Here's how the part is built. I have some questions about the finished solid (model axes, mm). A direction names the side the tool comes from. Round coordinates to 2 decimals unless told otherwise and drop trailing zeros. Write each loop counter-clockwise with the first axis right and the second up, starting at its lowest first coordinate (ties: lowest second). Pieces come first, ordered by that corner, then holes. Notation, with made-up numbers: (69, 10) -> (81, 10) arc R12 ccw to (81, 19) -> close; hole circle Ø4 at (-28.5, 63.5). An arc over 180 degrees is marked (long way). Put each result on its own line as item: value. Start each with the question number.
1. Suppose I cut it at C-C (x = 0). Please give me the cut outline in (y, z), then the cut area to 3 significant figures.
2. For pin 1 (1.6 mm diameter, centred on x = 0, y = 0, fed in from -Z); pin 2 (1 mm diameter, centred on y = -2, z = 4.5, fed in from -X); pin 3 (2 mm diameter, centred on x = 2, y = 0.5, fed in from +Z), each with a flat end and sliding along its axis, tell me the tip position at first contact or that it passes through.
3. Which directions (+Z, -Z, +X, -X, +Y, -Y) give clear straight access to the entire face, cutting with the end or side of a thin tool? Please do faces 4 (the face through (5.1, -2.14, 5.06)), 5 (the face through (-1.2, -0.9, 4)), 6 (the face through (-3, 1, 2)).
4. Suppose I cut it at A-A (x = -2.25). Please give me the cut outline in (y, z).
5. I need wall thicknesses on probe 1 along Y at (x, z) = (0, 1.15); probe 2 along Z at (x, y) = (-0.25, -1.5); probe 3 along X at (y, z) = (0, 8.5). Which ranges of each line are inside material? Lowest first, please. Write a range as from..to.
6. We'd pull the mould along X, two halves only. Please class faces 1 (the face through (0, 1.4, 2)), 2 (the face through (-5.14, 2.1, 5.06)), 3 (the face through (-1.2, -0.9, 0)): +X half, -X half, draft (parallel to the pull), parting line (faces both ways), or undercut.
```python
from build123d import *

# Parameters (mm, degrees)
F0_W         = 12
F0_H         = 6
F0_W_2       = 10.4
F0_H_2       = 4.4
F1_DEPTH     = 9
F2_R         = 2.19999
F3_R         = 2.99999
F4_DEPTH     = 4
F5_T4_DEPTH  = 19
F5_S5_R      = 2.99999
F5_T6_DEPTH  = 11
F5_T10_DEPTH = 19
F5_S11_R     = 2.99999
F5_T12_DEPTH = 11
F5_T16_DEPTH = 19
F5_S17_R     = 2.99999
F5_T18_DEPTH = 11
F5_T22_DEPTH = 19
F5_S23_R     = 2.99999
F5_T24_DEPTH = 11
F6_R         = 1


# Not quite as in the source:
# - a fillet or chamfer that OpenCascade refuses, or shapes differently, is made with other operations: its cross-section is extruded or revolved along the edge and cut away or added
# - a fillet or chamfer is up to 0.001 mm smaller than in the source, because OpenCascade refuses the exact size


with BuildPart() as f1:
    # F0 (on Top) → F1 (new body)
    with BuildSketch(Plane.XY):
        Rectangle(F0_W, F0_H)
        Rectangle(F0_W_2, F0_H_2, mode=Mode.SUBTRACT)
    extrude(amount=F1_DEPTH)

    # F2 (radius 2.2 in the source; OpenCascade refuses exactly that, so slightly less here)
    f2_edges = [f1.edges().sort_by_distance(p)[0] for p in [
        (-5.2, 2.2, 4.5),
        (-5.2, -2.2, 4.5),
        (5.2, 2.2, 4.5),
        (5.2, -2.2, 4.5),
    ]]
    fillet(f2_edges, radius=F2_R)

    # F3 (radius 3 in the source; OpenCascade refuses exactly that, so slightly less here)
    f3_edges = [f1.edges().sort_by_distance(p)[0] for p in [
        (-6, 3, 4.5),
        (6, 3, 4.5),
        (-6, -3, 4.5),
        (6, -3, 4.5),
    ]]
    fillet(f3_edges, radius=F3_R)

    # F0 (on Top) → F4 (join)
    with BuildSketch(Plane.XY):
        Rectangle(F0_W_2, F0_H_2)
        with BuildLine():
            Line((-0.9069178574, 1), (-4.4, 1))
            Line((-4.4, 1), (-4.4, 1.4))
            Line((-4.4, 1.4), (4.4, 1.4))
            Line((4.4, 1.4), (4.4, 1))
            Line((4.4, 1), (0.9069178574, 1))
            ThreePointArc((0.9069178574, 1), (1.2342688336, 0.5468824794), (1.35, 0))
            ThreePointArc((1.35, 0), (-0.5468824794, -1.2342688336), (-0.9069178574, 1))
        make_face(mode=Mode.SUBTRACT)
    extrude(amount=F4_DEPTH)

    # F5: fillet of radius 3 on 4 edges, made by hand


with BuildPart() as f5_tool2:
    # F5_s3 → F5_t4 (new body)
    with BuildSketch(Plane.XY.offset(-7.5)):
        with BuildLine():
            ThreePointArc((-2.2, -2.2), (-4.3213203436, -1.3213203436), (-5.2, 0.8))
            Line((-5.2, 0.8), (-5.2, -2.2))
            Line((-5.2, -2.2), (-2.2, -2.2))
        make_face()
    extrude(amount=F5_T4_DEPTH)

    # F5_s5 → F5_t6 (cut, symmetric)
    with BuildSketch(Plane.XY.offset(2)):
        with Locations((-3.00001, -1e-05)):
            Circle(F5_S5_R)
    extrude(amount=F5_T6_DEPTH, both=True, mode=Mode.SUBTRACT)


with BuildPart() as f1_1:
    add(f1.part)

    # F5_t1: cut F5_tool2
    add(f5_tool2.part, mode=Mode.SUBTRACT)


with BuildPart() as f5_tool8:
    # F5_s9 → F5_t10 (new body)
    with BuildSketch(Plane.XY.offset(-7.5)):
        with BuildLine():
            ThreePointArc((5.2, 0.8), (4.3213203436, -1.3213203436), (2.2, -2.2))
            Line((2.2, -2.2), (5.2, -2.2))
            Line((5.2, -2.2), (5.2, 0.8))
        make_face()
    extrude(amount=F5_T10_DEPTH)

    # F5_s11 → F5_t12 (cut, symmetric)
    with BuildSketch(Plane.XY.offset(2)):
        with Locations((3.00001, -1e-05)):
            Circle(F5_S11_R)
    extrude(amount=F5_T12_DEPTH, both=True, mode=Mode.SUBTRACT)


with BuildPart() as f1_2:
    add(f1_1.part)

    # F5_t7: cut F5_tool8
    add(f5_tool8.part, mode=Mode.SUBTRACT)


with BuildPart() as f5_tool14:
    # F5_s15 → F5_t16 (new body)
    with BuildSketch(Plane.XY.offset(-7.5)):
        with BuildLine():
            ThreePointArc((-5.2, -0.8), (-4.3213203436, 1.3213203436), (-2.2, 2.2))
            Line((-2.2, 2.2), (-5.2, 2.2))
            Line((-5.2, 2.2), (-5.2, -0.8))
        make_face()
    extrude(amount=F5_T16_DEPTH)

    # F5_s17 → F5_t18 (cut, symmetric)
    with BuildSketch(Plane.XY.offset(2)):
        with Locations((-3.00001, 1e-05)):
            Circle(F5_S17_R)
    extrude(amount=F5_T18_DEPTH, both=True, mode=Mode.SUBTRACT)


with BuildPart() as f1_3:
    add(f1_2.part)

    # F5_t13: cut F5_tool14
    add(f5_tool14.part, mode=Mode.SUBTRACT)


with BuildPart() as f5_tool20:
    # F5_s21 → F5_t22 (new body)
    with BuildSketch(Plane.XY.offset(-7.5)):
        with BuildLine():
            ThreePointArc((5.2, -0.8), (4.3213203436, 1.3213203436), (2.2, 2.2))
            Line((2.2, 2.2), (5.2, 2.2))
            Line((5.2, 2.2), (5.2, -0.8))
        make_face()
    extrude(amount=F5_T22_DEPTH)

    # F5_s23 → F5_t24 (cut, symmetric)
    with BuildSketch(Plane.XY.offset(2)):
        with Locations((3.00001, 1e-05)):
            Circle(F5_S23_R)
    extrude(amount=F5_T24_DEPTH, both=True, mode=Mode.SUBTRACT)


with BuildPart() as f1_4:
    add(f1_3.part)

    # F5_t19: cut F5_tool20
    add(f5_tool20.part, mode=Mode.SUBTRACT)

    # F6
    f6_edges = [f1_4.edges().sort_by_distance(p)[0] for p in [
        (0, -3, 0),
    ]]
    fillet(f6_edges, radius=F6_R)


solid = f1_4.part
```
Verdict:
1. outline: (-3, 1) arc R1 ccw to (-2, 0) -> (-1.35, 0) -> (-1.35, 4) -> (-2.2, 4) -> (-2.2, 9) -> (-3, 9) -> close; (1.4, 0) -> (2, 0) arc R1 ccw to (3, 1) -> (3, 9) -> (2.2, 9) -> (2.2, 4) -> (1.4, 4) -> close
1. area: 20.6 mm^2
2. pin 1: passes through
2. pin 2: stops at x = -5.6
2. pin 3: stops at z = 4
3. face 4: +Z, -Z, +X, -Y
3. face 5: +Z
3. face 6: +Z, -Z
4. outline: (-3, 1) arc R1 ccw to (-2, 0) -> (1, 0) -> (1, 4) -> (-2.2, 4) -> (-2.2, 9) -> (-3, 9) -> close; (1.4, 0) -> (2, 0) arc R1 ccw to (3, 1) -> (3, 9) -> (2.2, 9) -> (2.2, 4) -> (1.4, 4) -> close
5. probe 1: y = -3..-1.35, 1.4..3
5. probe 2: z = 0..4
5. probe 3: x = -6..-5.2, 5.2..6
6. face 1: undercut
6. face 2: -X half
6. face 3: draft
